Geometry check sheet. Reference: the model listing, model coordinates, mm. A direction names the side the tool comes from. Round coordinates to 2 decimals unless told otherwise and drop trailing zeros. Return JSON: item names as keys, results as strings. Group by question number.
from build123d import *

# Parameters (mm, degrees)
CUT_EXTRUDE1_DEPTH      = 86.356590332
CUT_EXTRUDE1_DEPTH_BACK = 86.356590332
SKETCH9_R               = 28.237117721
BOSS_EXTRUDE3_DEPTH     = 4.5
SKETCH10_R              = 28.237117721
SKETCH10_R_2            = 27.47603731
CUT_EXTRUDE2_DEPTH      = 0.5
CUT_EXTRUDE4_DEPTH      = 0.5
CUT_EXTRUDE5_DEPTH      = 0.5
BOSS_EXTRUDE5_DEPTH     = 0.5
CUT_EXTRUDE7_DEPTH      = 0.5
CUT_EXTRUDE7_DEPTH_BACK = 0.5
SKETCH11_11_R           = 5
SKETCH11_12_R           = 0.5
CUT_EXTRUDE8_DEPTH      = 0.5


with BuildPart() as part:
    # Sketch1 → Revolve1 (revolve)
    with BuildSketch(Plane.XY):
        with BuildLine():
            Line((0, 49.509049853), (0, -35))
            Line((0, -35), (-25.272030651, -35))
            ThreePointArc((-25.272030651, -35), (-47.186298393, 17.586623254), (0, 49.509049853))
        make_face()
    revolve(axis=Axis((0, 0, 0), (0, 1, 0)))

    # Sketch2 → Cut-Extrude1 (cut, two sides: drawn at the far end of the back side and taken through both)
    with BuildSketch(Plane.XY.offset(-CUT_EXTRUDE1_DEPTH_BACK)):
        Polygon((57.527772065, 42), (57.527772065, 50), (-10, 50), (-49.614603295, 50), (-49.614603295, 42), align=None)
    extrude(amount=CUT_EXTRUDE1_DEPTH + CUT_EXTRUDE1_DEPTH_BACK, mode=Mode.SUBTRACT)

    # Sketch8 → Revolve2 (revolve)
    with BuildSketch(Plane.XY, mode=Mode.PRIVATE) as revolve2_sk:
        Polygon((-29.237117721, 42), (-29.237117721, 46), (-28.237117721, 46.5), (-28.237117721, 42), align=None)
    revolve(revolve2_sk.sketch.rotate(Axis((0, 0, 0), (0, 1, 0)), 270), axis=Axis((0, 0, 0), (0, 1, 0)))

    # Sketch9 → Boss-Extrude3 (add)
    with BuildSketch(Plane(origin=(0, 42, 0), x_dir=(1, 0, 0), z_dir=(0, 1, 0))):
        Circle(SKETCH9_R)
    extrude(amount=BOSS_EXTRUDE3_DEPTH)

    # Sketch10 → Cut-Extrude2 (cut)
    with BuildSketch(Plane(origin=(0, 46.5, 0), x_dir=(1, 0, 0), z_dir=(0, 1, 0))):
        with Locations(Location((0, 0, 0), (0, 0, 270))):
            Circle(SKETCH10_R)
        with Locations(Location((0, 0, 0), (0, 0, 270))):
            Circle(SKETCH10_R_2, mode=Mode.SUBTRACT)
    extrude(amount=-CUT_EXTRUDE2_DEPTH, mode=Mode.SUBTRACT)

    # Sketch11 → Cut-Extrude4 (cut)
    with BuildSketch(Plane(origin=(0, 46.5, 0), x_dir=(1, 0, 0), z_dir=(0, 1, 0))):
        with BuildLine():
            Line((-2.662439007, -12.315535384), (-6.158792876, -12.315535384))
            ThreePointArc((-6.158792876, -12.315535384), (-7.326955988, -13.483698497), (-6.158792876, -14.651861609))
            Line((-6.158792876, -14.651861609), (-2.662439007, -14.651861609))
            ThreePointArc((-2.662439007, -14.651861609), (-1.494275894, -13.483698497), (-2.662439007, -12.315535384))
        make_face()
    extrude(amount=-CUT_EXTRUDE4_DEPTH, mode=Mode.SUBTRACT)

    # Sketch11_7 → Cut-Extrude5 (cut)
    with BuildSketch(Plane(origin=(0, 46.5, 0), x_dir=(1, 0, 0), z_dir=(0, 1, 0))):
        with BuildLine():
            Line((2.662439007, -12.315535384), (6.158792876, -12.315535384))
            ThreePointArc((6.158792876, -12.315535384), (7.326955988, -13.483698497), (6.158792876, -14.651861609))
            Line((6.158792876, -14.651861609), (2.662439007, -14.651861609))
            ThreePointArc((2.662439007, -14.651861609), (1.494275894, -13.483698497), (2.662439007, -12.315535384))
        make_face()
    extrude(amount=-CUT_EXTRUDE5_DEPTH, mode=Mode.SUBTRACT)

    # Sketch11_10 → Boss-Extrude5 (add)
    with BuildSketch(Plane(origin=(0, 46.5, 0), x_dir=(1, 0, 0), z_dir=(0, 1, 0))):
        with BuildLine():
            Line((9.284761758, 10.683638038), (-9.284761758, 10.683638038))
            ThreePointArc((-9.284761758, 10.683638038), (-12.820295664, 9.219171944), (-14.284761758, 5.683638038))
            Line((-14.284761758, 5.683638038), (-14.284761758, -4.367615893))
            ThreePointArc((-14.284761758, -4.367615893), (-12.820295664, -7.903149799), (-9.284761758, -9.367615893))
            Line((-9.284761758, -9.367615893), (9.284761758, -9.367615893))
            ThreePointArc((9.284761758, -9.367615893), (12.820295664, -7.903149799), (14.284761758, -4.367615893))
            Line((14.284761758, -4.367615893), (14.284761758, 5.683638038))
            ThreePointArc((14.284761758, 5.683638038), (12.820295664, 9.219171944), (9.284761758, 10.683638038))
        make_face()
    extrude(amount=BOSS_EXTRUDE5_DEPTH)

    # Sketch11_11 → Cut-Extrude7 (cut, two sides: drawn at the far end of the back side and taken through both)
    with BuildSketch(Plane(origin=(0, 46.5, 0), x_dir=(1, 0, 0), z_dir=(0, 1, 0)).offset(-CUT_EXTRUDE7_DEPTH_BACK)):
        with Locations(Location((0, 0, 0), (0, 0, 270))):
            Circle(SKETCH11_11_R)
    extrude(amount=CUT_EXTRUDE7_DEPTH + CUT_EXTRUDE7_DEPTH_BACK, mode=Mode.SUBTRACT)

    # Sketch11_12 → Cut-Extrude8 (cut)
    with BuildSketch(Plane(origin=(0, 46.5, 0), x_dir=(1, 0, 0), z_dir=(0, 1, 0))):
        with Locations(Location((0, 23.265511796, 0), (0, 0, 270))):
            Circle(SKETCH11_12_R)
    extrude(amount=-CUT_EXTRUDE8_DEPTH, mode=Mode.SUBTRACT)


solid = part.part
1. Mould release check, pull along X, two halves, no side actions. Record for faces 5 (the face through (8.25, 46.25, 26.21)), 6 (the face through (11.198, 44.028, -27.008)), 7 (the face through (-12.78, 46.75, -9.26)): pulls with the +X half, pulls with the -X half, needs draft (parallel to the pull), parting line crosses it, or undercut.
2. Depth check by flat-ended pin: pin 1 Ø8 at (x, y) = (-24.5, 3) entering from +Z; pin 2 Ø2 at (y, z) = (-24.5, 27) entering from +X; pin 3 Ø0.6 at (x, y) = (-5.5, 46.5) entering from +Z. Enter the tip coordinate at first touch or a pass-through.
3. Tool access check on faces 1 (the face through (12.781, 46.746, 7.942)), 2 (the face through (-27.566, 46.254, -6.121)), 3 (the face through (-12.859, 46.746, 7.864)), 4 (the face through (12.86, 46.75, -9.18)). Record the directions out of +Z, -Z, +X, -X, +Y, -Y that give a thin tool (end or side, any length) a straight path to the whole face; none if there is none.
4. Material ranges on line 1 along Y through (x, z) = (-23, 1.5); line 2 along Z through (x, y) = (24, 5.5); line 3 along X through (y, z) = (31, -27), recorded low to high.
Result sheet:
{
 "1": {"face 5": "undercut", "face 6": "parting line crosses it", "face 7": "pulls with the -X half"},
 "2": {"pin 1": "stops at z = 44.56", "pin 2": "stops at x = 28.69", "pin 3": "stops at z = 28.31"},
 "3": {"face 1": "+Z, +X, +Y", "face 2": "+Y", "face 3": "+Z, -X, +Y", "face 4": "-Z, +X, +Y"},
 "4": {"line 1": "y = -35 to 46.5", "line 2": "z = -42.8 to 42.8", "line 3": "x = -30.3 to 30.3"}
}
